Verification items for the finished model (mm, model axes). Face numbers are marked on the shaded views. Round coordinates to 2 decimals unless told otherwise and drop trailing zeros. Loops run counter-clockwise (first coordinate to the right, second up) from the corner with the lowest first, then second, coordinate; pieces in that order, holes last. Notation, with made-up numbers: (25, -2.75) - (33, -2.75) arc R12 cw to (33, 15.25) - close; hole circle Ø4 at (25, 61). An arc over 180 degrees is marked (long way). Use a Markdown table: item, result. Add a question column.
Autodesk Inventor part; units mm, degrees
ref_plane "YZ Plane" through (0, 0, 0) normal (1, 0, 0) x (0, 1, 0)
ref_plane "XY Plane" through (0, 0, 0) normal (0, 0, 1) x (1, 0, 0)
sketch "Skizze1" plane through (0, 0, 0) normal (0, 1, 0) x (-1, 0, 0)
  line L0 (0, 0) -> (0, -2.8868)
  line L1 (0, -2.8868) -> (-2.5, -4.3301)
  line L2 (-2.5, -4.3301) -> (-5, -2.8868)
  line L3 (-5, -2.8868) -> (-5, 0)
  line L4 (-5, 0) -> (-2.5, 1.4434)
  line L5 (-2.5, 1.4434) -> (0, 0)
  dimension "d2" = 120
  dimension "d4" = 120
  dimension "d6" = 120
  dimension "d8" = 120
  dimension "d11" = 5
  dimension "d12" = 5
  dimension "d13" = 5
extrude "Extrusion1" add sketch "Skizze1" along normal blind 26
sketch "Skizze2" plane through (0, 26, 0) normal (0, 1, 0) x (1, 0, 0)
  line L0 (0, 2.8868) -> (0, 0)
  line L1 (5, 0) -> (5, 2.8868)
  line L2 (0, 0) -> (5, 2.8868) construction
  line L3 (0, 2.8868) -> (5, 0) construction
  point P0 (2.5, 1.4434)
hole "Bohrung1" at (2.5, 26, -1.4434) direction (0, -1, 0) diameter 3 end through all
thread "Gewinde1"
properties part number "abstandshalter_26mm"
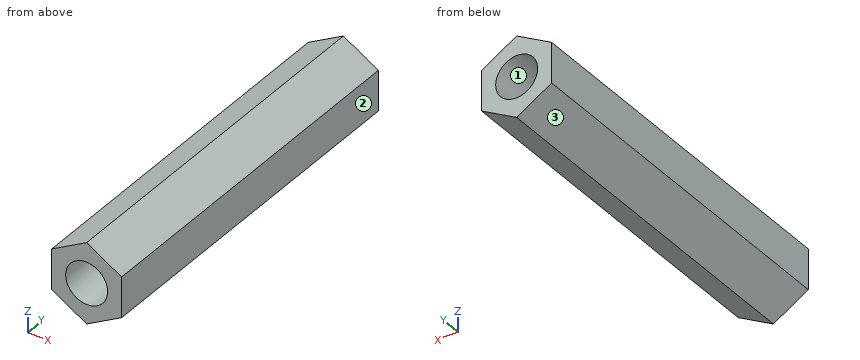
Q1. Release check for a two-part mould opening along Z. For the marked faces 1, 2 and 3 record: +Z half, -Z half, draft (parallel to the pull), parting line (faces both ways), or undercut.
Q2. Section check B-B on y = 2. Record the cut outline in (x, z).
Q3. Thickness scan on line 1 along X through (y, z) = (11.25, -1.4); line 2 along X through (y, z) = (6.25, -2.45); line 3 along Z through (x, y) = (3.3, 1.75). Record the ranges inside material, lowest first.
Q4. Go/stop test with flat-tipped pins: pin 1 Ø1.5 at (x, y) = (1.5, 12.5) entering from -Z; pin 2 Ø1 at (x, y) = (0.5, 18.5) entering from -Z; pin 3 Ø1 at (y, z) = (4, 0) entering from -X; pin 4 Ø1.5 at (x, y) = (4, 7) entering from -Z. Record where each tip stops, or that it passes through.
Q5. Section check D-D on x = 0.5. Record the cut outline in (y, z), plus the area to 3 significant figures.
Q6. Section check C-C on z = -1.4. Record the cut outline in (x, y), plus the area to 3 significant figures.
Q7. Section check A-A on x = 3.1. Record the cut outline in (y, z).
Determined:
| question | item | result |
|---|---|---|
| 1 | face 1 | undercut |
| 1 | face 2 | draft |
| 1 | face 3 | -Z half |
| 2 | outline | (0, -2.89) - (2.5, -4.33) - (5, -2.89) - (5, 0) - (2.5, 1.44) - (0, 0) - close; hole circle Ø3 at (2.5, -1.44) |
| 3 | line 1 | x = 0 to 1, 4 to 5 |
| 3 | line 2 | x = 0 to 1.39, 3.61 to 5 |
| 3 | line 3 | z = -3.87 to -2.71, -0.17 to 0.98 |
| 4 | pin 1 | stops at z = -4.19 |
| 4 | pin 2 | stops at z = -3.46 |
| 4 | pin 3 | stops at x = 0 |
| 4 | pin 4 | stops at z = -3.9 |
| 5 | outline | (0, -3.18) - (26, -3.18) - (26, 0.29) - (0, 0.29) - close |
| 5 | area | 90.1 mm² |
| 6 | outline | (0, 0) - (1, 0) - (1, 26) - (0, 26) - close; (4, 0) - (5, 0) - (5, 26) - (4, 26) - close |
| 6 | area | 52.0 mm² |
| 7 | outline | (0, -3.98) - (26, -3.98) - (26, -2.82) - (0, -2.82) - close; (0, -0.07) - (26, -0.07) - (26, 1.1) - (0, 1.1) - close |
